Here's how the part is built. I have some questions about the finished solid (model axes, mm). A direction names the side the tool comes from. Round coordinates to 2 decimals unless told otherwise and drop trailing zeros. Write each loop counter-clockwise with the first axis right and the second up, starting at its lowest first coordinate (ties: lowest second). Pieces come first, ordered by that corner, then holes. Notation, with made-up numbers: M 89.25,1 L 131.25,1 A25 ccw 131.25,28 Z; hole C 87,16.25 d5. An arc over 180 degrees is marked long. Use a Markdown table: item, result. Add a question column.
```python
from build123d import *

# Parameters (mm, degrees)
SKETCH1_R           = 154.626985005
BOSS_EXTRUDE1_DEPTH = 38.1
BOSS_EXTRUDE2_START = -38.1
SKETCH2_R           = 124.46
BOSS_EXTRUDE2_DEPTH = 69.3
SKETCH3_R           = 139.7
CUT_EXTRUDE1_DEPTH  = 6.35
FILLET1_R           = 6.35


with BuildPart() as part:
    # Sketch1 → Boss-Extrude1 (new body)
    with BuildSketch(Plane(origin=(0, 0, 0), x_dir=(0, 0, -1), z_dir=(1, 0, 0))):
        with Locations(Location((0, 0, 0), (0, 0, 180))):
            Circle(SKETCH1_R)
    extrude(amount=BOSS_EXTRUDE1_DEPTH)

    # Sketch2 → Boss-Extrude2 (add)
    with BuildSketch(Plane(origin=(38.1, 0, 0), x_dir=(0, 0, -1), z_dir=(1, 0, 0)).offset(BOSS_EXTRUDE2_START)):
        Circle(SKETCH2_R)
    extrude(amount=BOSS_EXTRUDE2_DEPTH)

    # Sketch3 → Cut-Extrude1 (cut)
    with BuildSketch(Plane.ZY):
        Circle(SKETCH3_R)
    extrude(amount=-CUT_EXTRUDE1_DEPTH, mode=Mode.SUBTRACT)

    # Fillet1
    fillet1_edges = [part.edges().sort_by_distance(p)[0] for p in [
        (0, 0, -154.626985005),
    ]]
    fillet(fillet1_edges, radius=FILLET1_R)


solid = part.part
```
Item 1: If we mould it in two halves opening along Y, with no side actions, what happens to faces 4 (the face through (22, -130.4, 83.1)), 5 (the face through (6.35, 2, -2)), 6 (the face through (69.3, 2, 2))? For each: +Y half, -Y half, draft (parallel to the pull), parting line (faces both ways), or undercut.
Item 2: On a 3-axis mill with a long thin cutter (end or side, diameter ignored), from which of +Z, -Z, +X, -X, +Y, -Y can I reach the whole of each face in a straight line? I mean faces 1 (the face through (38.1, -69, -104)), 2 (the face through (0, 100, 100)), 3 (the face through (3.13, -85.01, -110.86)). Say none if no direction works.
Item 3: I need wall thicknesses on probe 1 along X at (y, z) = (-79.5, 32.5); probe 2 along X at (y, z) = (103, -100); probe 3 along Y at (x, z) = (5.25, 0). Which ranges of each line are inside material? Lowest first, please. Write a range as from..to.
Item 4: Imagine slicing it at D-D on x = 49.5. List the corners of the cut face in (y, z) for me, plus the area to 3 significant figures.
Item 5: Imagine slicing it at C-C on x = 28.5. List the corners of the cut face in (y, z) for me.
Item 6: Imagine slicing it at A-A on z = 0. List the corners of the cut face in (x, y) for me.
Item 7: For pin 1 Ø4 at (x, y) = (24, 12.5) entering from +Z; pin 2 Ø4 at (x, y) = (45, 49) entering from -Z; pin 3 Ø1.5 at (x, y) = (33, -73) entering from -Z, each with a flat end and sliding along its axis, tell me the tip position at first contact or that it passes through.
The answers:
| question | item | result |
|---|---|---|
| 1 | face 4 | parting line |
| 1 | face 5 | undercut |
| 1 | face 6 | draft |
| 2 | face 1 | +X |
| 2 | face 2 | +Z, -Z, -X, +Y, -Y |
| 2 | face 3 | -X |
| 3 | probe 1 | 6.35..69.3 |
| 3 | probe 2 | 0..38.1 |
| 3 | probe 3 | -154.53..-139.7, 139.7..154.53 |
| 4 | outline | C 0,0 d248.92 |
| 4 | area | 48,700 mm² |
| 5 | outline | C 0,0 d309.25 |
| 6 | outline | M 0,-148.28 A6.35 ccw 6.35,-154.63 L 38.1,-154.63 L 38.1,-124.46 L 69.3,-124.46 L 69.3,124.46 L 38.1,124.46 L 38.1,154.63 L 6.35,154.63 A6.35 ccw 0,148.28 L 0,139.7 L 6.35,139.7 L 6.35,-139.7 L 0,-139.7 Z |
| 7 | pin 1 | z = 154.27 |
| 7 | pin 2 | z = -115.24 |
| 7 | pin 3 | z = -136.71 |
